```python
from build123d import *

# Parameters (mm, degrees)
F0_R     = 5
F1_DEPTH = 2
F2_D     = 9
F3_R     = 2


with BuildPart() as f1:
    # F0 (on Top) → F1 (new body)
    with BuildSketch(Plane.XY):
        Polygon((0, -8.0829037687), (7, -4.0414518843), (7, 4.0414518843), (0, 8.0829037687), (-7, 4.0414518843), (-7, -4.0414518843), align=None)
        Circle(F0_R, mode=Mode.SUBTRACT)
        Circle(F0_R)
    extrude(amount=F1_DEPTH)

    # F2 (through all)
    with Locations(Plane(origin=(0, 0, 0), x_dir=(1, 0, 0), z_dir=(0, 0, -1))):
        with Locations((0, 0)):
            Hole(F2_D / 2)

    # F3
    f3_edges = [f1.edges().sort_by_distance(p)[0] for p in [
        (0, -8.082904, 1),
        (7, -4.041452, 1),
        (7, 4.041452, 1),
        (0, 8.082904, 1),
        (-7, 4.041452, 1),
        (-7, -4.041452, 1),
    ]]
    fillet(f3_edges, radius=F3_R)


solid = f1.part
```
Geometry check sheet. Reference: the model listing, model coordinates, mm. Round coordinates to 2 decimals unless told otherwise and drop trailing zeros. Write each loop counter-clockwise with the first axis right and the second up, starting at its lowest first coordinate (ties: lowest second). Pieces come first, ordered by that corner, then holes. Notation, with made-up numbers: (55, 34.25) - (73, 34.25) arc R36 cw to (73, 72.25) - close; hole circle Ø7 at (86.25, 77.25). An arc over 180 degrees is marked (long way). Write each question's results on one line, items separated by ' | '.
(1) Thickness scan on probe 1 along Y at (x, z) = (0, 0.65); probe 2 along X at (y, z) = (1.5, 0.15); probe 3 along X at (y, z) = (3, 0.9). Record the ranges inside material, lowest first. Write a range as from..to.
Computed:
probe 1: y = -7.77..-4.5, 4.5..7.77 | probe 2: x = -7..-4.24, 4.24..7 | probe 3: x = -7..-3.35, 3.35..7
(2) Sectioned sample at A-A, the plane y = 0. Enter the section's corners in (x, z), plus the area to 3 significant figures.
Computed:
outline: (-7, 0) - (-4.5, 0) - (-4.5, 2) - (-7, 2) - close; (4.5, 0) - (7, 0) - (7, 2) - (4.5, 2) - close | area: 10.0 mm^2
(3) Sectioned sample at C-C, the plane z = 0.9. Enter the section's corners in (x, y), plus the area to 3 significant figures.
Computed:
outline: (-7, -2.89) arc R2 ccw to (-6, -4.62) - (-1, -7.51) arc R2 ccw to (1, -7.51) - (6, -4.62) arc R2 ccw to (7, -2.89) - (7, 2.89) arc R2 ccw to (6, 4.62) - (1, 7.51) arc R2 ccw to (-1, 7.51) - (-6, 4.62) arc R2 ccw to (-7, 2.89) - close; hole circle Ø9 at (0, 0) | area: 105 mm^2
(4) Draft check along X on faces 1 (the face through (0.015, -7.773, 1.014)), 2 (the face through (0.59, -4.46, 1.01)), 3 (the face through (7, 0, 1)), 4 (the face through (-7, 0, 1)). Enter one of: pulls with the +X half, pulls with the -X half, needs draft (parallel to the pull), parting line crosses it, or undercut.
Computed:
face 1: parting line crosses it | face 2: undercut | face 3: pulls with the +X half | face 4: pulls with the -X half
(5) Sectioned sample at D-D, the plane y = 6.25. Enter the section's corners in (x, z), plus the area to 3 significant figures.
Computed:
outline: (-3.17, 0) - (3.17, 0) - (3.17, 2) - (-3.17, 2) - close | area: 12.7 mm^2
(6) Sectioned sample at B-B, the plane x = 0. Enter the section's corners in (y, z), plus the area to 3 significant figures.
Computed:
outline: (-7.77, 0) - (-4.5, 0) - (-4.5, 2) - (-7.77, 2) - close; (4.5, 0) - (7.77, 0) - (7.77, 2) - (4.5, 2) - close | area: 13.1 mm^2
